Geometry: see drawing. Coordinates: mm, zero at the bounding-box minimum. Round coordinates to 2 decimals unless told otherwise and drop trailing zeros. Order: outer loops, then holes, each group sorted by start corner. A loop starts at its lowest first (then second) coordinate and runs counter-clockwise, first axis right, second up. Notation, with made-up numbers: (88, 79) - (127, 79) arc R26 cw to (127, 102) - close; hole circle Ø4 at (-30.75, 36). An arc over 180 degrees is marked (long way). Put each result on its own line as item: value. Start each with the question number.
1) Section A-A on x = 50.8. Output: boundary loops of the cut face in (y, z), then the cut area to 3 significant figures.
2) Section C-C on y = 15.5. Output: boundary loops of the cut face in (x, z), then the cut area to 3 significant figures.
3) Mould query, pull axis Y, two halves, no side actions, for the marked faces 1, 2 and 3. Classes: +Y half, -Y half, draft (parallel to the pull), parting line (faces both ways), or undercut.
4) Section B-B on z = 188.5. Output: boundary loops of the cut face in (x, y), then the cut area to 3 significant figures.
5) Contact query for flat-ended pins moving along their axis: P1, Ø4, axis at y = 21.5, z = 134, coming from the -X side; P2, Ø1, axis at y = 16, z = 119, coming from the +X side; P3, Ø14, axis at x = 8.5, y = 6.5, coming from the +Z side; P4, Ø2, axis at x = 16.5, y = 16.5, coming from the +Z side. Output: stop coordinate, or through.
6) Section D-D on z = 84. Output: boundary loops of the cut face in (x, y), then the cut area to 3 significant figures.
7) Line query: probe 1 along X at (y, z) = (22.25, 215.9); probe 2 along Z at (x, y) = (54.5, 21.25); probe 3 along Y at (x, z) = (54, 78). Output: solid intervals per line, ascending. Write a range as [from, to].
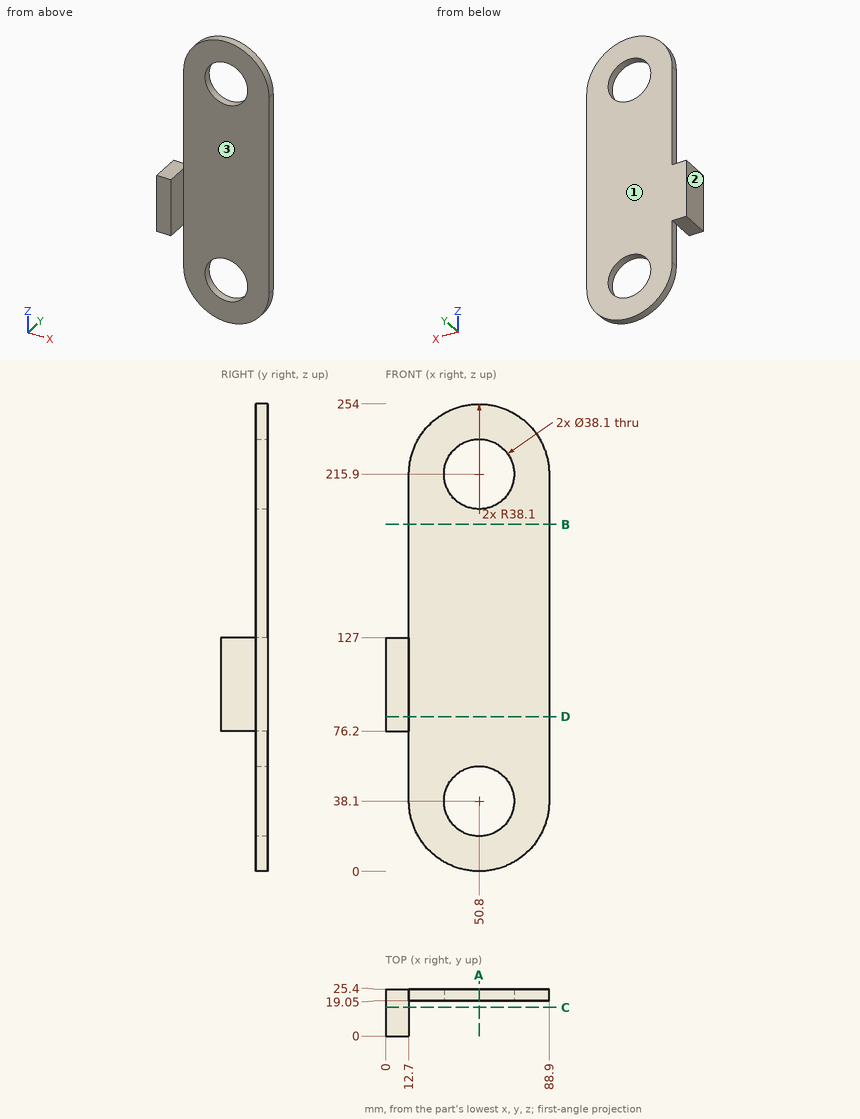
Answer sheet:
1. outline: (19.05, 0) - (25.4, 0) - (25.4, 19.05) - (19.05, 19.05) - close; (19.05, 57.15) - (25.4, 57.15) - (25.4, 196.85) - (19.05, 196.85) - close; (19.05, 234.95) - (25.4, 234.95) - (25.4, 254) - (19.05, 254) - close
1. area: 1,130 mm^2
2. outline: (0, 76.2) - (12.7, 76.2) - (12.7, 127) - (0, 127) - close
2. area: 645 mm^2
3. face 1: +Y half
3. face 2: draft
3. face 3: -Y half
4. outline: (12.7, 19.05) - (88.9, 19.05) - (88.9, 25.4) - (12.7, 25.4) - close
4. area: 484 mm^2
5. P1: x = 12.7
5. P2: x = 12.7
5. P3: z = 127
5. P4: through
6. outline: (0, 0) - (12.7, 0) - (12.7, 19.05) - (88.9, 19.05) - (88.9, 25.4) - (0, 25.4) - close
6. area: 806 mm^2
7. probe 1: [12.7, 31.75], [69.85, 88.9]
7. probe 2: [0.18, 19.41], [56.79, 197.21], [234.59, 253.82]
7. probe 3: [19.05, 25.4]
